```python
from build123d import *

# Parameters (mm, degrees)
SKETCH1_W                                           = 155.7
SKETCH1_H                                           = 155.7
BOSS_EXTRUDE2_DEPTH                                 = 80
SKETCH3_W                                           = 8
SKETCH3_H                                           = 25
BOSS_EXTRUDE4_DEPTH                                 = 145.45
CHAMFER1_SIZE                                       = 0.508
CHAMFER1_SIZE2                                      = 0.03552282
CHAMFER2_SIZE                                       = 0.508
CHAMFER2_SIZE2                                      = 0.03552282
SKETCH4_W                                           = 8.2
SKETCH4_H                                           = 25.2
CUT_EXTRUDE6_DEPTH                                  = 160.2
FILLET1_R                                           = 1
SKETCH6_W                                           = 10.35
SKETCH6_H                                           = 10.25
CUT_EXTRUDE7_DEPTH                                  = 80
SKETCH7_W                                           = 10.25
SKETCH7_H                                           = 10.25
BOSS_EXTRUDE5_DEPTH                                 = 80
CSK_FOR_M3_COUNTERSUNK_FLAT_HEAD_SCREW1_D           = 3.4
CSK_FOR_M3_COUNTERSUNK_FLAT_HEAD_SCREW1_DEPTH       = 16
CSK_FOR_M3_COUNTERSUNK_FLAT_HEAD_SCREW1_CSINK_D     = 6.3
CSK_FOR_M3_COUNTERSUNK_FLAT_HEAD_SCREW1_CSINK_ANGLE = 90
CSK_FOR_M3_COUNTERSUNK_FLAT_HEAD_SCREW1_TIP         = 1.021463052
SKETCH12_R                                          = 2.1
CUT_EXTRUDE9_DEPTH                                  = 5
FILLET2_START                                       = -18.821212121
FILLET2_DEPTH                                       = 152.821212121
FILLET3_START                                       = -18.821212121
FILLET3_DEPTH                                       = 152.821212121
SKETCH14_W                                          = 9.8
SKETCH14_H                                          = 9.8
BOSS_EXTRUDE6_DEPTH                                 = 8
CUT_EXTRUDE12_START                                 = -9.8
SKETCH17_W                                          = 6
SKETCH17_H                                          = 1
CUT_EXTRUDE12_DEPTH                                 = 1
CUT_EXTRUDE13_START                                 = -9.8
SKETCH19_W                                          = 6
SKETCH19_H                                          = 1
CUT_EXTRUDE13_DEPTH                                 = 1
BOSS_EXTRUDE7_DEPTH                                 = 5
BOSS_EXTRUDE7_DEPTH_BACK                            = 80
SKETCH20_W                                          = 25
SKETCH20_H                                          = 25
SKETCH21_W                                          = 20.8
SKETCH21_H                                          = 20.8
BOSS_EXTRUDE8_DEPTH                                 = 38
SKETCH23_W                                          = 12.85
SKETCH23_H                                          = 12.85
CUT_EXTRUDE14_DEPTH                                 = 38
CSK_FOR_M4_COUNTERSUNK_FLAT_HEAD_SCREW1_D           = 4.5
CSK_FOR_M4_COUNTERSUNK_FLAT_HEAD_SCREW1_DEPTH       = 26
CSK_FOR_M4_COUNTERSUNK_FLAT_HEAD_SCREW1_CSINK_D     = 9.4
CSK_FOR_M4_COUNTERSUNK_FLAT_HEAD_SCREW1_CSINK_ANGLE = 90
CSK_FOR_M4_COUNTERSUNK_FLAT_HEAD_SCREW1_TIP         = 1.351936393


with BuildPart() as part:
    # Sketch1 → Boss-Extrude2 (new body)
    with BuildSketch(Plane(origin=(0, 0, 0), x_dir=(1, 0, 0), z_dir=(0, 1, 0))):
        with Locations((55.528787879, -61.975)):
            Rectangle(SKETCH1_W, SKETCH1_H)
    extrude(amount=BOSS_EXTRUDE2_DEPTH)

    # Sketch3 → Boss-Extrude4 (add)
    with BuildSketch(Plane.XY.offset(-15.875)):
        with Locations((137.378787879, 40)):
            Rectangle(SKETCH3_W, SKETCH3_H)
    extrude(amount=BOSS_EXTRUDE4_DEPTH)

    # Chamfer1
    chamfer1_edges = [part.edges().sort_by_distance(p)[0] for p in [
        (141.378787879, 52.5, 56.85),
    ]]
    chamfer1_side = [part.faces().sort_by_distance(p)[0] for p in [
        (137.378787879, 52.5, 56.85),
    ]]
    chamfer(chamfer1_edges, length=CHAMFER1_SIZE, length2=CHAMFER1_SIZE2, reference=chamfer1_side[0])

    # Chamfer2
    chamfer2_edges = [part.edges().sort_by_distance(p)[0] for p in [
        (141.378787879, 27.5, 56.85),
    ]]
    chamfer2_side = [part.faces().sort_by_distance(p)[0] for p in [
        (137.378787879, 27.5, 56.85),
    ]]
    chamfer(chamfer2_edges, length=CHAMFER2_SIZE, length2=CHAMFER2_SIZE2, reference=chamfer2_side[0])

    # Sketch4 → Cut-Extrude6 (cut)
    with BuildSketch(Plane.ZY.offset(-141.378787879)):
        with Locations((-11.775, 40)):
            Rectangle(SKETCH4_W, SKETCH4_H)
    extrude(amount=CUT_EXTRUDE6_DEPTH, mode=Mode.SUBTRACT)

    # Fillet1
    fillet1_edges = [part.edges().sort_by_distance(p)[0] for p in [
        (141.378787879, 40, -7.675),
    ]]
    fillet(fillet1_edges, radius=FILLET1_R)

    # Sketch6 → Cut-Extrude7 (cut)
    with BuildSketch(Plane(origin=(0, 80, 0), x_dir=(1, 0, 0), z_dir=(0, 1, 0))):
        with Locations((128.203787879, -134.7)):
            Rectangle(SKETCH6_W, SKETCH6_H)
    extrude(amount=-CUT_EXTRUDE7_DEPTH, mode=Mode.SUBTRACT)

    # Sketch7 → Boss-Extrude5 (add)
    with BuildSketch(Plane(origin=(0, 80, 0), x_dir=(1, 0, 0), z_dir=(0, 1, 0))):
        with Locations((-17.196212121, 21)):
            Rectangle(SKETCH7_W, SKETCH7_H)
    extrude(amount=-BOSS_EXTRUDE5_DEPTH)

    # CSK for M3 Countersunk Flat Head Screw1
    with Locations(Plane.ZY.offset(22.321212121)):
        with Locations((-21, 40)):
            CounterSinkHole(CSK_FOR_M3_COUNTERSUNK_FLAT_HEAD_SCREW1_D / 2, CSK_FOR_M3_COUNTERSUNK_FLAT_HEAD_SCREW1_CSINK_D / 2, depth=CSK_FOR_M3_COUNTERSUNK_FLAT_HEAD_SCREW1_DEPTH, counter_sink_angle=CSK_FOR_M3_COUNTERSUNK_FLAT_HEAD_SCREW1_CSINK_ANGLE)
            with Locations((0, 0, -(CSK_FOR_M3_COUNTERSUNK_FLAT_HEAD_SCREW1_DEPTH + CSK_FOR_M3_COUNTERSUNK_FLAT_HEAD_SCREW1_TIP / 2))):  # 118° drill point
                Cone(0, CSK_FOR_M3_COUNTERSUNK_FLAT_HEAD_SCREW1_D / 2, CSK_FOR_M3_COUNTERSUNK_FLAT_HEAD_SCREW1_TIP, mode=Mode.SUBTRACT)

    # Sketch12 → Cut-Extrude9 (cut)
    with BuildSketch(Plane.XY.offset(129.575)):
        with Locations((128.203787879, 40)):
            Circle(SKETCH12_R)
    extrude(amount=-CUT_EXTRUDE9_DEPTH, mode=Mode.SUBTRACT)

    # Fillet2: read off the stored shape, not the designer's step
    # Fillet2 outline → Fillet2 (cut)
    with BuildSketch(Plane.YZ.offset(FILLET2_START)):
        with BuildLine():
            Line((52.6, -15.875), (53.6, -15.875))
            ThreePointArc((53.6, -15.875), (52.892893219, -15.582106781), (52.6, -14.875))
            Line((52.6, -14.875), (52.6, -15.875))
        make_face()
    extrude(amount=FILLET2_DEPTH, mode=Mode.SUBTRACT)

    # Fillet3: read off the stored shape, not the designer's step
    # Fillet3 outline → Fillet3 (cut)
    with BuildSketch(Plane.YZ.offset(FILLET3_START)):
        with BuildLine():
            ThreePointArc((27.4, -14.875), (27.107106781, -15.582106781), (26.4, -15.875))
            Line((26.4, -15.875), (27.4, -15.875))
            Line((27.4, -15.875), (27.4, -14.875))
        make_face()
    extrude(amount=FILLET3_DEPTH, mode=Mode.SUBTRACT)

    # Sketch14 → Boss-Extrude6 (add)
    with BuildSketch(Plane(origin=(0, 80, 0), x_dir=(1, 0, 0), z_dir=(0, 1, 0))):
        with Locations((34.878787879, -82.625)):
            Rectangle(SKETCH14_W, SKETCH14_H)
    extrude(amount=BOSS_EXTRUDE6_DEPTH)

    # Sketch17 → Cut-Extrude12 (cut)
    with BuildSketch(Plane(origin=(39.778787879, 0, 0), x_dir=(0, 0, -1), z_dir=(1, 0, 0)).offset(CUT_EXTRUDE12_START)):
        with Locations((-82.625, 85.5)):
            Rectangle(SKETCH17_W, SKETCH17_H)
    extrude(amount=CUT_EXTRUDE12_DEPTH, mode=Mode.SUBTRACT)

    # Sketch19 → Cut-Extrude13 (cut)
    with BuildSketch(Plane(origin=(0, 0, 77.725), x_dir=(-1, 0, 0), z_dir=(0, 0, -1)).offset(CUT_EXTRUDE13_START)):
        with Locations((-34.878787879, 85.5)):
            Rectangle(SKETCH19_W, SKETCH19_H)
    extrude(amount=CUT_EXTRUDE13_DEPTH, mode=Mode.SUBTRACT)

    # Sketch20 → Boss-Extrude7 (add, two sides: drawn at the far end of the back side and taken through both)
    with BuildSketch(Plane(origin=(0, 0, 0), x_dir=(-1, 0, 0), z_dir=(0, -1, 0)).offset(-BOSS_EXTRUDE7_DEPTH_BACK)):
        with Locations((14.071212121, -131.575)):
            Rectangle(SKETCH20_W, SKETCH20_H)
    extrude(amount=BOSS_EXTRUDE7_DEPTH + BOSS_EXTRUDE7_DEPTH_BACK)

    # Sketch21 → Boss-Extrude8 (add)
    with BuildSketch(Plane(origin=(0, 80, 0), x_dir=(1, 0, 0), z_dir=(0, 1, 0))):
        with Locations((-14.071212121, -131.575)):
            Rectangle(SKETCH21_W, SKETCH21_H)
    extrude(amount=BOSS_EXTRUDE8_DEPTH)

    # Sketch23 → Cut-Extrude14 (cut)
    with BuildSketch(Plane(origin=(0, 118, 0), x_dir=(1, 0, 0), z_dir=(0, 1, 0))):
        with Locations((-14.071212121, -131.575)):
            Rectangle(SKETCH23_W, SKETCH23_H)
    extrude(amount=-CUT_EXTRUDE14_DEPTH, mode=Mode.SUBTRACT)

    # CSK for M4 Countersunk Flat Head Screw1
    with Locations(Plane.XY.offset(141.975)):
        with Locations((-14.071212121, 105)):
            CounterSinkHole(CSK_FOR_M4_COUNTERSUNK_FLAT_HEAD_SCREW1_D / 2, CSK_FOR_M4_COUNTERSUNK_FLAT_HEAD_SCREW1_CSINK_D / 2, depth=CSK_FOR_M4_COUNTERSUNK_FLAT_HEAD_SCREW1_DEPTH, counter_sink_angle=CSK_FOR_M4_COUNTERSUNK_FLAT_HEAD_SCREW1_CSINK_ANGLE)
            with Locations((0, 0, -(CSK_FOR_M4_COUNTERSUNK_FLAT_HEAD_SCREW1_DEPTH + CSK_FOR_M4_COUNTERSUNK_FLAT_HEAD_SCREW1_TIP / 2))):  # 118° drill point
                Cone(0, CSK_FOR_M4_COUNTERSUNK_FLAT_HEAD_SCREW1_D / 2, CSK_FOR_M4_COUNTERSUNK_FLAT_HEAD_SCREW1_TIP, mode=Mode.SUBTRACT)


solid = part.part
```
CAD build for the part. Positions are in the model's coordinates, mm. A direction names the side the tool comes from. Round coordinates to 2 decimals unless told otherwise and drop trailing zeros. Order: outer loops, then holes, each group sorted by start corner. A loop starts at its lowest first (then second) coordinate and runs counter-clockwise, first axis right, second up. Notation, with made-up numbers: (-2.75, 38.25) -> (11.25, 38.25) arc R32 ccw to (11.25, 70.25) -> close; hole circle Ø2 at (84, 63). An arc over 180 degrees is marked (long way). One line per question, with ' | ' between items.
Q1. Slice it at A-A (y = 105). Write the cut outline in (x, z) (3 decimals).
Completed:
outline: (-24.471, 121.175) -> (-16.321, 121.175) -> (-16.321, 125.15) -> (-20.496, 125.15) -> (-20.496, 138) -> (-16.321, 138) -> (-16.321, 139.525) -> (-18.771, 141.975) -> (-24.471, 141.975) -> close; (-11.821, 121.175) -> (-3.671, 121.175) -> (-3.671, 141.975) -> (-9.371, 141.975) -> (-11.821, 139.525) -> (-11.821, 138) -> (-7.646, 138) -> (-7.646, 125.15) -> (-11.821, 125.15) -> close
Q2. Probe probe 1 along Y at (x, z) = (51, -11.5); probe 2 along Z at (x, y) = (-19, 40) (3 decimals); probe 3 along Y at (x, z) = (-18, -21). List the from-to ranges inside material, lowest first.
Completed:
probe 1: y = 0 to 27.4, 52.6 to 80 | probe 2: z = -26.125 to -22.7, -19.3 to 144.075 | probe 3: y = 0 to 38.3, 41.7 to 80
Q3. Slice it at C-C (x = 120.5). Write the cut outline in (y, z) (3 decimals).
Completed:
outline: (0, -15.875) -> (26.4, -15.875) arc R1 ccw to (27.4, -14.875) -> (27.4, -7.675) -> (52.6, -7.675) -> (52.6, -14.875) arc R1 ccw to (53.6, -15.875) -> (80, -15.875) -> (80, 139.825) -> (0, 139.825) -> close
Q4. Slice it at D-D (z = 73). Write the cut outline in (x, y).
Completed:
outline: (-22.32, 0) -> (133.38, 0) -> (133.38, 27.5) -> (140.87, 27.5) -> (141.38, 27.54) -> (141.38, 52.46) -> (140.87, 52.5) -> (133.38, 52.5) -> (133.38, 80) -> (-22.32, 80) -> close
Q5. Two-plate mould, pull along Y, no slides. Class faces 1 (the flat face through (128, 40, 124.575)), 2 (the flat face through (35, 84, 77.725)), 3 (the flat face through (-21, 118, 131)): released by +Y, released by -Y, zero draft, split by the parting line, or undercut.
Completed:
face 1: undercut | face 2: zero draft | face 3: released by +Y
Q6. Which spindle directions (+Z, -Z, +X, -X, +Y, -Y) get a long thin tool onto all of the face, cutting with end or side? Do faces 4 (the flat face through (-14, 99, 141.975)), 5 (the flat face through (60, 13, -15.875)), 6 (the flat face through (137, 27.5, 60)). Say none if no direction does.
Completed:
face 4: +Z, +X, -X, +Y | face 5: -Z, +X, +Y, -Y | face 6: +Z, -Z, +X, -Y
Q7. Slice it at B-B (y = 92). Write the cut outline in (x, z) (3 decimals), then the cut area to 3 significant figures.
Completed:
outline: (-24.471, 121.175) -> (-3.671, 121.175) -> (-3.671, 141.975) -> (-24.471, 141.975) -> close; hole (-20.496, 125.15) -> (-7.646, 125.15) -> (-7.646, 138) -> (-20.496, 138) -> close | area: 268 mm^2
Q8. Drop flat-ended pins along their axis: pin 1 (0.5 mm diameter, centred on y = 85.5, z = 87, fed in from -X); pin 2 (10 mm diameter, centred on x = 23, y = 49, fed in from -Z) (3 decimals); pin 3 (8 mm diameter, centred on x = 54.5, z = 16.5, fed in from +Y); pin 4 (12 mm diameter, centred on x = 97.5, y = 87.5, fed in from +Z). Give the stop position or say it passes through.
Completed:
pin 1: stops at x = 29.98 | pin 2: stops at z = -15.875 | pin 3: stops at y = 80 | pin 4: passes through
